```python
from build123d import *

# Parameters (mm, degrees)
F1_DEPTH  = 22.352
F2_DEPTH  = 3.175
F3_R      = 10.922
F5_DEPTH  = 9.652
F6_DEPTH  = 9.652
F8_R      = 3.175
F9_DEPTH  = 22.352
F8_R_2    = 6.35
F10_DEPTH = 3.175


with BuildPart() as f1:
    # F0 (on Front) → F1 (new body, symmetric)
    with BuildSketch(Plane.XZ):
        Polygon((-8.0358399709, 0), (-33.4358399709, 0), (-52.4858399709, 32.9955678842), (-60.5815056276, 27.632467684), (-39.0553081737, -9.652), (30.0641600291, -9.652), (30.0641600291, 0), align=None)
    extrude(amount=F1_DEPTH, both=True)

    # F0 (on Front) → F2 (join, symmetric)
    with BuildSketch(Plane.XZ):
        Polygon((-52.4858399709, 32.9955678842), (-33.4358399709, 0), (-8.0358399709, 0), align=None)
    extrude(amount=F2_DEPTH, both=True)

    # F3
    f3_edges = [f1.edges().sort_by_distance(p)[0] for p in [
        (-56.533673, -22.352, 30.314018),
        (-56.533673, 22.352, 30.314018),
    ]]
    fillet(f3_edges, radius=F3_R)

    # F4 (on face) → F5 (join)
    with BuildSketch(Plane.XY):
        with BuildLine():
            Line((30.0641600291, -9.652), (30.0641600291, -22.352))
            ThreePointArc((30.0641600291, -22.352), (52.4161600291, 0), (30.0641600291, 22.352))
            Line((30.0641600291, 22.352), (30.0641600291, 9.652))
            ThreePointArc((30.0641600291, 9.652), (39.7161600291, 0), (30.0641600291, -9.652))
        make_face()
    extrude(amount=-F5_DEPTH)

    # F4 (on face) → F6 (cut)
    with BuildSketch(Plane.XY):
        with BuildLine():
            Line((4.6641600291, -9.652), (30.0641600291, -9.652))
            Line((30.0641600291, -9.652), (30.0641600291, 0))
            Line((30.0641600291, 0), (30.0641600291, 9.652))
            Line((30.0641600291, 9.652), (4.6641600291, 9.652))
            ThreePointArc((4.6641600291, 9.652), (-4.9878399709, 0), (4.6641600291, -9.652))
        make_face()
    extrude(amount=-F6_DEPTH, mode=Mode.SUBTRACT)

    # F8 (on face) → F9 (cut)
    with BuildSketch(Plane(origin=(-25.0768799782, 0, -14.4781434058), x_dir=(0, 1, 0), z_dir=(0.8660254038, 0, 0.5))):
        with Locations((-11.417399453, 42.3558945687)):
            Circle(F8_R)
        with Locations((11.4397590045, 42.816884833)):
            Circle(F8_R)
    extrude(amount=-F9_DEPTH, mode=Mode.SUBTRACT)

    # F8 (on face) → F10 (cut)
    with BuildSketch(Plane(origin=(-25.0768799782, 0, -14.4781434058), x_dir=(0, 1, 0), z_dir=(0.8660254038, 0, 0.5))):
        with Locations((-11.417399453, 42.3558945687)):
            Circle(F8_R_2)
        with Locations((-11.417399453, 42.3558945687)):
            Circle(F8_R, mode=Mode.SUBTRACT)
        with Locations((11.4397590045, 42.816884833)):
            Circle(F8_R_2)
        with Locations((11.4397590045, 42.816884833)):
            Circle(F8_R, mode=Mode.SUBTRACT)
    extrude(amount=-F10_DEPTH, mode=Mode.SUBTRACT)


solid = f1.part
```
Model file for the job. Use its own axes, mm. A direction names the side the tool comes from. Coordinates: 2 decimals unless noted, no trailing zeros. Loops run counter-clockwise (first coordinate to the right, second up) from the corner with the lowest first, then second, coordinate; pieces in that order, holes last. Notation, with made-up numbers: (-5, -5.75) -> (4, -5.75) arc R16 ccw to (4, 7.25) -> close; hole circle Ø9 at (32.25, -30.75). An arc over 180 degrees is marked (long way). Answer as a JSON object with one key per item and string values.
Q1. Cut at B-B (x = 17). List the corners of the cut face in (y, z).
Report:
{"outline": "(-22.35, -9.65) -> (-9.65, -9.65) -> (-9.65, 0) -> (-22.35, 0) -> close; (9.65, -9.65) -> (22.35, -9.65) -> (22.35, 0) -> (9.65, 0) -> close"}
Q2. Cut at C-C (x = -3). List the corners of the cut face in (y, z), and give its area (3 significant figures).
Report:
{"outline": "(-22.35, -9.65) -> (-5.87, -9.65) -> (-5.87, 0) -> (-22.35, 0) -> close; (5.87, -9.65) -> (22.35, -9.65) -> (22.35, 0) -> (5.87, 0) -> close", "area": "318 mm2"}
Q3. 3-axis set-ups, long thin cutter, end or side, ignore diameter. For faces 4 (the flat face through (-40.71, 12.63, 12.6)), 5 (the flat face through (9, 10, 0)), 6 (the flat face through (-15.9, -22.352, -0.4)), 7 (the flat face through (-47.64, -8.68, 18.25)), 8 (the flat face through (18, 9.652, -5)): which of +Z, -Z, +X, -X, +Y, -Y reach the whole face in a straight line?
Report:
{"face 4": "+Z, +X, +Y", "face 5": "+Z, +X", "face 6": "+Z, -Z, +X, -X, -Y", "face 7": "none", "face 8": "+Z, -Z"}
Q4. Cut at D-D (z = 19.5). State how many separate pieces and enclosed holes the cut face has, and give its area (3 significant figures).
Report:
{"separate pieces": "3", "enclosed holes": "0", "area": "392 mm2"}
Q5. Pull direction Z, two halves, no side cores. Call faces 1 (the flat face through (-56.48, -0.16, 30.35)), 2 (the flat face through (-30, 3.175, 10)), 3 (the flat face through (-47.87, 14.17, 18.65)): released by +Z, released by -Z, zero draft, split by the parting line, or undercut.
Report:
{"face 1": "released by +Z", "face 2": "zero draft", "face 3": "undercut"}
Q6. Probe probe 1 along Z at (x, y) = (11.5, 11); probe 2 along Y at (x, z) = (-37, 16.5) (3 decimals); probe 3 along X at (y, z) = (4, 15.5). List the from-to ranges inside material, lowest first.
Report:
{"probe 1": "z = -9.65 to 0", "probe 2": "y = -3.175 to 3.175", "probe 3": "x = -53.58 to -42.38"}
Q7. Flat gauge pins, fed straight in: P1, Ø12, axis at y = -11.5, z = 9.5, coming from the +X side; P2, Ø10, axis at y = 12.5, z = 1.5, coming from the +X side; P3, Ø10, axis at x = -29.5, z = 20.5, coming from the +Y side (3 decimals); P4, Ø12, axis at x = -12, z = 1, coming from the -Y side. Where does each tip first touch, or does it go through?
Report:
{"P1": "stops at x = -35.46", "P2": "stops at x = 51.04", "P3": "stops at y = 3.175", "P4": "stops at y = -22.35"}
Q8. Cut at A-A (y = 0). List the corners of the cut face in (x, z).
Report:
{"outline": "(-60.58, 27.63) -> (-39.06, -9.65) -> (-4.99, -9.65) -> (-4.99, 0) -> (-8.04, 0) -> (-52.49, 33) -> close; (39.72, -9.65) -> (52.42, -9.65) -> (52.42, 0) -> (39.72, 0) -> close"}
